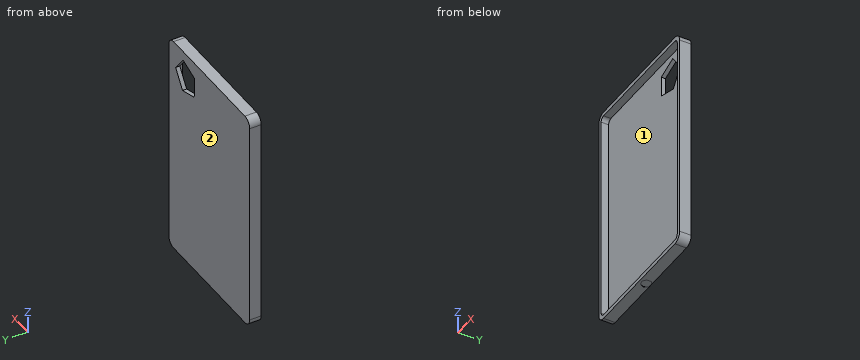
```python
from build123d import *

# Parameters (mm, degrees)
F0_W     = 85.0665410506
F0_H     = 138.3
F1_DEPTH = 7.1
F2_R     = 5.08
F3_T     = -2.54
F5_DEPTH = 25
F8_DEPTH = 0.1


# Not quite as in the source:
# - a feature of the source that left no trace in its solid (it failed there, or was rolled back) is left out


with BuildPart() as f1:
    # F0 (on Front) → F1 (new body)
    with BuildSketch(Plane.XZ):
        Rectangle(F0_W, F0_H)
    extrude(amount=F1_DEPTH)

    # F2
    f2_edges = [f1.edges().sort_by_distance(p)[0] for p in [
        (42.533271, -3.55, -69.15),
        (-42.533271, -3.55, -69.15),
        (42.533271, -3.55, 69.15),
        (-42.533271, -3.55, 69.15),
    ]]
    fillet(f2_edges, radius=F2_R)

    # F3
    f3_openings = [f1.faces().sort_by_distance(p)[0] for p in [
        (0, -7.1, 0),
    ]]
    offset(amount=F3_T, openings=f3_openings)

    # F4 (on face) → F5 (cut)
    with BuildSketch(Plane.XZ.offset(2.54)):
        Polygon((15.775061698, 46.2421439753), (28.0853956244, 42.6747929635), (35.2822504398, 53.2802441743), (27.4198174015, 63.4021245005), (15.3637117341, 59.0523393613), align=None)
    extrude(amount=-F5_DEPTH, mode=Mode.SUBTRACT)

    # F7 (on face) → F8 (cut)
    with BuildSketch(Plane(origin=(0, 0, -69.15), x_dir=(1, 0, 0), z_dir=(0, 0, -1))):
        Polygon((2.8688537423, 1.343842895), (2.8688537423, 4.1069771897), (0.7085483604, 5.8297632436), (-1.9853083886, 5.2149080197), (-3.1841874281, 2.7254100423), (-1.9853083886, 0.235912065), (0.7085483604, -0.3789431589), align=None)
    extrude(amount=-F8_DEPTH, mode=Mode.SUBTRACT)


solid = f1.part
```
The listing builds one solid part. Answer for the finished solid, in the listing's coordinates (mm). Face numbers are marked on the shaded views. A direction names the side the tool comes from. Give positions to 0.01 mm unless a question says otherwise; leave off trailing zeros. Write each loop counter-clockwise with the first axis right and the second up, starting at its lowest first coordinate (ties: lowest second). Pieces come first, ordered by that corner, then holes. Notation, with made-up numbers: (-15.75, -39) -> (-8.75, -39) arc R15 cw to (-8.75, -14) -> close; hole circle Ø10 at (63.5, 56.5). An arc over 180 degrees is marked (long way). Write item = value, one per line. Start each with the question number.
1) The part is cut by section A-A, the plane x = 33. Determine the outline of the cut face in (y, z).
2) Which of the six approach directions +Z, -Z, +X, -X, +Y, -Y give full straight-line access (tool end or side, diameter ignored) to the marked faces 1 and 2?
3) The part is cut by section C-C, the plane x = -8.5. Determine the outline of the cut face in (y, z).
4) Straight lines are drawn through the part: line 1 along X through (y, z) = (-6, -61); line 2 along Z through (x, y) = (21.5, -3.75); line 3 along Y through (x, z) = (13, -14). For each, find the intervals that lie inside material, in ascending order.
5) This flat-tipped pin is pushed along its axis until it touches: pin 1 (3 mm diameter, centred on x = 5.5, z = -49.5, fed in from -Y). Where does it stop, or does it pass through?
6) The part is cut by section D-D, the plane z = 55. Determine the outline of the cut face in (x, y), and give its area (3 significant figures).
7) The part is cut by section B-B, the plane z = 9. Determine the outline of the cut face in (x, y), and give its area (3 significant figures).
Solutions:
q1.outline = (-7.1, -69.15) -> (0, -69.15) -> (0, 49.92) -> (-2.54, 49.92) -> (-2.54, -66.61) -> (-7.1, -66.61) -> close; (-7.1, 66.61) -> (-2.54, 66.61) -> (-2.54, 56.22) -> (0, 56.22) -> (0, 69.15) -> (-7.1, 69.15) -> close
q2.face_1 = -Y
q2.face_2 = +Z, -Z, +X, -X, +Y
q3.outline = (-7.1, -69.15) -> (0, -69.15) -> (0, 69.15) -> (-7.1, 69.15) -> (-7.1, 66.61) -> (-2.54, 66.61) -> (-2.54, -66.61) -> (-7.1, -66.61) -> close
q4.line_1 = -42.53 to -39.99, 39.99 to 42.53
q4.line_2 = -69.15 to -66.61, 66.61 to 69.15
q4.line_3 = -2.54 to 0
q5.pin_1 = -2.54
q6.outline = (-42.53, -7.1) -> (-39.99, -7.1) -> (-39.99, -2.54) -> (15.49, -2.54) -> (15.49, 0) -> (-42.53, 0) -> close; (33.95, -2.54) -> (39.99, -2.54) -> (39.99, -7.1) -> (42.53, -7.1) -> (42.53, 0) -> (33.95, 0) -> close
q6.area = 192 mm²
q7.outline = (-42.53, -7.1) -> (-39.99, -7.1) -> (-39.99, -2.54) -> (39.99, -2.54) -> (39.99, -7.1) -> (42.53, -7.1) -> (42.53, 0) -> (-42.53, 0) -> close
q7.area = 239 mm²
